Check sheet for the modelled part. Datum: model origin and axes. Units: mm. A direction names the side the tool comes from. Round coordinates to 2 decimals unless told otherwise and drop trailing zeros. Loops run counter-clockwise (first coordinate to the right, second up) from the corner with the lowest first, then second, coordinate; pieces in that order, holes last. Notation, with made-up numbers: (38.5, 16.25) - (88.5, 16.25) arc R12 cw to (88.5, 29.25) - close; hole circle Ø2 at (-2, 71). An arc over 180 degrees is marked (long way). Put each result on its own line as item: value. Start each with the question number.
Item 1: Tool access check on faces 5 (the flat face through (3, 86.325, 0)), 6 (the flat face through (44, 108.46, 0)), 7 (the flat face through (123, 86.713, 0)). Record the directions out of +Z, -Z, +X, -X, +Y, -Y that give a thin tool (end or side, any length) a straight path to the whole face; none if there is none.
Item 2: Section check B-B, the plane x = -8. Record the cut outline in (y, z), and give its area (3 significant figures).
Item 3: Section check A-A, the plane y = 5. Record the cut outline in (x, z), and give its area (3 significant figures).
Item 4: Draft check along Y on faces 1 (the cylindrical face through (-80.998, 111.126, 0.07)), 2 (the flat face through (56.8, 97.8, 0.1)), 3 (the flat face through (-3, 92, 5)), 4 (the flat face through (-12.365, 52.444, 0.07)). Enter one of: pulls with the +Y half, pulls with the -Y half, needs draft (parallel to the pull), parting line crosses it, or undercut.
Item 5: Section check C-C, the plane y = 100. Record the cut outline in (x, z).
Item 6: Section check D-D, the plane y = 20. Record the cut outline in (x, z), and give its area (3 significant figures).
Item 7: Material ranges on line 1 along Y through (x, z) = (-6.5, 0); line 2 along X through (y, z) = (104, 4); line 3 along Y through (x, z) = (-16, -4), recorded low to high.
Item 8: Gauge pin test, flat ends, axial feed: pin 1 Ø22 at (x, y) = (-54.69, 96.71) entering from -Z; pin 2 Ø5 at (y, z) = (62, -1.5) entering from -X; pin 3 Ø5 at (x, z) = (121.5, 2) entering from -Y; pin 4 Ø6 at (y, z) = (40, -2.5) entering from +X. Record the tip position at first contact, or that the pin passes through.
from build123d import *

# Parameters (mm, degrees)
SKETCH1_R           = 9.5
BOSS_EXTRUDE2_DEPTH = 5
SKETCH2_R           = 2
CUT_EXTRUDE1_DEPTH  = 43.5


with BuildPart() as part:
    # Sketch1 → Boss-Extrude2 (new, symmetric)
    with BuildSketch(Plane.XY):
        with BuildLine():
            Line((-25, 0), (0, 0))
            Line((0, 0), (0, 34.32666264))
            Line((0, 34.32666264), (-25.081844034, 71.075487971))
            ThreePointArc((-25.081844034, 71.075487971), (-26.228666022, 80.106897872), (-19.579322507, 86.325241404))
            Line((-19.579322507, 86.325241404), (26.604717255, 86.325241404))
            ThreePointArc((26.604717255, 86.325241404), (27.367190328, 86.423753026), (28.079588429, 86.712818196))
            Line((28.079588429, 86.712818196), (66.87872037, 86.712818196))
            ThreePointArc((66.87872037, 86.712818196), (67.591118471, 86.423753026), (68.353591544, 86.325241404))
            Line((68.353591544, 86.325241404), (114.623497212, 86.325241404))
            ThreePointArc((114.623497212, 86.325241404), (115.385970286, 86.423753026), (116.098368387, 86.712818196))
            Line((116.098368387, 86.712818196), (130, 86.712818196))
            Line((130, 86.712818196), (122.946920772, 126.712818196))
            Line((122.946920772, 126.712818196), (-54.687026413, 126.712818196))
            ThreePointArc((-54.687026413, 126.712818196), (-81.213991187, 110.724247098), (-79.465738474, 79.800827522))
            Line((-79.465738474, 79.800827522), (-25, 0))
        make_face()
        with BuildLine():
            Line((-34.048206361, 32.250592263), (-44.320136127, 47.300576318))
            ThreePointArc((-44.320136127, 47.300576318), (-44.262816837, 50.76404185), (-40.978396488, 51.864706177))
            Line((-40.978396488, 51.864706177), (-17.56266475, 44.823773781))
            ThreePointArc((-17.56266475, 44.823773781), (-15.450916476, 42.332556513), (-16.865487004, 39.388981395))
            Line((-16.865487004, 39.388981395), (-30.009288975, 31.379929737))
            ThreePointArc((-30.009288975, 31.379929737), (-32.202518151, 31.009156908), (-34.048206361, 32.250592263))
        make_face(mode=Mode.SUBTRACT)
        with Locations((-54.687026413, 96.712818196)):
            Circle(SKETCH1_R, mode=Mode.SUBTRACT)
        with BuildLine():
            ThreePointArc((25.16023195, 102.779114733), (23.586428727, 106.151820228), (26.505685136, 108.460486719))
            Line((26.505685136, 108.460486719), (61.945496305, 108.460486719))
            ThreePointArc((61.945496305, 108.460486719), (64.78922159, 106.416115571), (63.757193592, 103.069304387))
            Line((63.757193592, 103.069304387), (49.637443167, 92.371369228))
            ThreePointArc((49.637443167, 92.371369228), (48.10033357, 91.775144389), (46.480292695, 92.081179573))
            Line((46.480292695, 92.081179573), (25.16023195, 102.779114733))
        make_face(mode=Mode.SUBTRACT)
    extrude(amount=BOSS_EXTRUDE2_DEPTH, both=True)

    # Sketch2 → Cut-Extrude1 (cut, symmetric)
    with BuildSketch(Plane(origin=(0, 0, 0), x_dir=(0, 0, -1), z_dir=(1, 0, 0))):
        with Locations(Location((0, 5, 0), (0, 0, 90))):
            Circle(SKETCH2_R)
        with Locations(Location((0, 20, 0), (0, 0, 90))):
            Circle(SKETCH2_R)
    extrude(amount=CUT_EXTRUDE1_DEPTH, both=True, mode=Mode.SUBTRACT)


solid = part.part
Check result:
1. face 5: +Z, -Z, +X
1. face 6: +Z, -Z
1. face 7: +Z, -Z, +X, -Y
2. outline: (0, -5) - (46.05, -5) - (46.05, 5) - (0, 5) - close; (86.33, -5) - (126.71, -5) - (126.71, 5) - (86.33, 5) - close; hole circle Ø4 at (5, 0); hole circle Ø4 at (20, 0)
2. area: 839 mm²
3. outline: (-28.41, -5) - (0, -5) - (0, -2) - (-28.41, -2) - close; (-28.41, 2) - (0, 2) - (0, 5) - (-28.41, 5) - close
3. area: 170 mm²
4. face 1: parting line crosses it
4. face 2: undercut
4. face 3: needs draft
4. face 4: undercut
5. outline: (-84.51, -5) - (-63.6, -5) - (-63.6, 5) - (-84.51, 5) - close; (-45.77, -5) - (30.7, -5) - (30.7, 5) - (-45.77, 5) - close; (59.71, -5) - (127.66, -5) - (127.66, 5) - (59.71, 5) - close
6. outline: (-38.65, -5) - (0, -5) - (0, -2) - (-38.65, -2) - close; (-38.65, 2) - (0, 2) - (0, 5) - (-38.65, 5) - close
6. area: 232 mm²
7. line 1: 0 to 3, 7 to 18, 22 to 43.85, 86.33 to 126.71
7. line 2: -83.79 to -60.78, -48.59 to 23.89, 64.57 to 126.95
7. line 3: 0 to 40.19, 43.71 to 57.77, 86.33 to 126.71
8. pin 1: z = -5
8. pin 2: x = -69.02
8. pin 3: y = 86.71
8. pin 4: x = -1.82
